Autodesk Inventor part; units mm, degrees
ref_plane "YZ Plane" through (0, 0, 0) normal (1, 0, 0) x (0, 1, 0)
ref_plane "XZ Plane" through (0, 0, 0) normal (0, 1, 0) x (-1, 0, 0)
ref_plane "XY Plane" through (0, 0, 0) normal (0, 0, 1) x (1, 0, 0)
sketch "Sketch1" plane through (0, 0, 0) normal (0, 0, 1) x (1, 0, 0)
  line L0 (0, 0) -> (20.32, 0)
  line L1 (20.32, 0) -> (20.32, -139.7)
  line L2 (20.32, -139.7) -> (0, -139.7)
  line L3 (0, -139.7) -> (0, 0)
  line L4 (0, 0) -> (7.62, 0)
  line L5 (20.32, 0) -> (12.7, 0)
  line L6 (7.62, 0) -> (7.62, -3.302)
  line L7 (12.7, 0) -> (12.7, -3.302)
  line L8 (12.7, -3.302) -> (17.78, -3.302)
  line L9 (17.78, -3.302) -> (17.78, -8.382)
  line L10 (17.78, -8.382) -> (12.7, -8.382)
  line L11 (12.7, -8.382) -> (12.7, -13.462)
  line L12 (12.7, -13.462) -> (7.62, -13.462)
  line L13 (7.62, -13.462) -> (7.62, -8.382)
  line L14 (7.62, -8.382) -> (2.54, -8.382)
  line L15 (2.54, -8.382) -> (2.54, -3.302)
  line L16 (2.54, -3.302) -> (7.62, -3.302)
  line L17 (7.62, -3.302) -> (7.62, 0)
  dimension "d0" = 20.32
  dimension "d1" = 139.7
  dimension "d2" = 7.62
  dimension "d3" = 7.62
  dimension "d4" = 3.302
  dimension "d5" = 5.08
  dimension "d6" = 5.08
  dimension "d7" = 5.08
  dimension "d8" = 5.08
  dimension "d9" = 5.08
  dimension "d10" = 5.08
  dimension "d11" = 5.08
  dimension "d12" = 5.08
  dimension "d13" = 5.08
extrude "Extrusion1" add sketch "Sketch1" along normal blind 13.97 contours L0 L6 L16 L15 L14 L13 L12 L11 L10 L9 L8 L7 L1 L2 L3
sketch "Sketch2" plane through (20.32, -139.7, 0) normal (1, 0, 0) x (0, 0, -1)
  line L0 (-10.7501, 15.4155) -> (-10.7501, 26.5915)
  line L1 (-10.7501, 26.5915) -> (-1.8601, 26.5915)
  line L2 (-1.8601, 26.5915) -> (-1.8601, 15.4155)
  line L3 (-1.8601, 15.4155) -> (-10.7501, 15.4155)
  line L4 (-10.7501, 65.6672) -> (-10.7501, 77.0972)
  line L5 (-10.7501, 77.0972) -> (-1.8601, 77.0972)
  line L6 (-1.8601, 77.0972) -> (-1.8601, 65.6672)
  line L7 (-1.8601, 65.6672) -> (-10.7501, 65.6672)
  point P0 (0, 139.7)
  dimension "d16" = 11.176
  dimension "d17" = 8.89
  dimension "d18" = 11.43
  dimension "d19" = 8.89
extrude "Extrusion2" cut sketch "Sketch2" against normal blind 533.4
shell "Shell1" thickness 6.35 removed faces 1 at (20.32, -20.8676, 8.24)
sketch "Sketch3" plane through (0, 0, 13.97) normal (0, 0, 1) x (1, 0, 0)
  point P0 (0, 0)
properties part number "ripnewvertical2"
Here's how the part is built. I have some questions about the finished solid (model axes, mm). A direction names the side the tool comes from. Give positions to 0.01 mm unless a question says otherwise; leave off trailing zeros. Write each loop counter-clockwise with the first axis right and the second up, starting at its lowest first coordinate (ties: lowest second). Pieces come first, ordered by that corner, then holes. Notation, with made-up numbers: (-40, 1) -> (-18, 1) arc R18 cw to (-18, 15) -> close; hole circle Ø6 at (52, 74). An arc over 180 degrees is marked (long way). Write each question's results on one line, items separated by ' | '.
Item 1: Suppose I cut it at B-B on z = 4.5. Write out the boundary of the cut face in (x, y).
Output:
outline: (0, -139.7) -> (20.32, -139.7) -> (20.32, -124.28) -> (0, -124.28) -> close; (0, -113.11) -> (20.32, -113.11) -> (20.32, -74.03) -> (0, -74.03) -> close; (0, -62.6) -> (20.32, -62.6) -> (20.32, 0) -> (12.7, 0) -> (12.7, -3.3) -> (17.78, -3.3) -> (17.78, -8.38) -> (12.7, -8.38) -> (12.7, -13.46) -> (7.62, -13.46) -> (7.62, -8.38) -> (2.54, -8.38) -> (2.54, -3.3) -> (7.62, -3.3) -> (7.62, 0) -> (0, 0) -> close
Item 2: Suppose I cut it at A-A on x = 15.75. Write out the boundary of the cut face in (y, z).
Output:
outline: (-139.7, 0) -> (-8.38, 0) -> (-8.38, 13.97) -> (-139.7, 13.97) -> close; (-3.3, 0) -> (0, 0) -> (0, 13.97) -> (-3.3, 13.97) -> close; hole (-133.35, 6.35) -> (-130.63, 6.35) -> (-130.63, 7.62) -> (-133.35, 7.62) -> close; hole (-124.28, 1.86) -> (-113.11, 1.86) -> (-113.11, 10.75) -> (-124.28, 10.75) -> close; hole (-106.76, 6.35) -> (-80.38, 6.35) -> (-80.38, 7.62) -> (-106.76, 7.62) -> close; hole (-74.03, 1.86) -> (-62.6, 1.86) -> (-62.6, 10.75) -> (-74.03, 10.75) -> close; hole (-56.25, 6.35) -> (-19.81, 6.35) -> (-19.81, 7.62) -> (-56.25, 7.62) -> close
Item 3: We'd pull the mould along X, two halves only. Please class faces 1 (the face through (7.62, -11, 7)), 2 (the face through (0, -71, 12)), 3 (the face through (2.54, -6, 7)), 4 (the face through (10, -139.7, 7)): pulls with the +X half, pulls with the -X half, needs draft (parallel to the pull), parting line crosses it, or undercut.
Output:
face 1: undercut | face 2: pulls with the -X half | face 3: undercut | face 4: needs draft
Item 4: If I drill on L1, parallel to Y at x = 16.25, z = 5.5; L2, parallel to Y at x = 1.75, z = 10.25; L3, parallel to Y at x = 12.25, z = 6, over which ranges is the centre line in solid material (lowest first)?
Output:
L1: y = -139.7 to -124.28, -113.11 to -74.03, -62.6 to -8.38, -3.3 to 0 | L2: y = -139.7 to -124.28, -113.11 to -74.03, -62.6 to 0 | L3: y = -139.7 to -124.28, -113.11 to -74.03, -62.6 to -13.46
Item 5: Suppose I cut it at D-D on x = 9. Write out the boundary of the cut face in (y, z), plus the area to 3 significant figures.
Output:
outline: (-139.7, 0) -> (-13.46, 0) -> (-13.46, 13.97) -> (-139.7, 13.97) -> close; hole (-133.35, 6.35) -> (-130.63, 6.35) -> (-130.63, 7.62) -> (-133.35, 7.62) -> close; hole (-124.28, 1.86) -> (-113.11, 1.86) -> (-113.11, 10.75) -> (-124.28, 10.75) -> close; hole (-106.76, 6.35) -> (-80.38, 6.35) -> (-80.38, 7.62) -> (-106.76, 7.62) -> close; hole (-74.03, 1.86) -> (-62.6, 1.86) -> (-62.6, 10.75) -> (-74.03, 10.75) -> close; hole (-56.25, 6.35) -> (-19.81, 6.35) -> (-19.81, 7.62) -> (-56.25, 7.62) -> close | area: 1,480 mm^2
Item 6: Suppose I cut it at C-C on y = -69. Write out the boundary of the cut face in (x, z).
Output:
outline: (0, 0) -> (20.32, 0) -> (20.32, 1.86) -> (0, 1.86) -> close; (0, 10.75) -> (20.32, 10.75) -> (20.32, 13.97) -> (0, 13.97) -> close
Item 7: For pin 1 Ø4 at (x, z) = (6.5, 11) entering from +Y; pin 2 Ø3 at (y, z) = (-64.5, 7.5) entering from -X; pin 3 Ø1 at (x, z) = (10, 6) entering from +Y, each with a flat end and sliding along its axis, tell me the tip position at first contact or that it passes through.
Output:
pin 1: stops at y = 0 | pin 2: passes through | pin 3: stops at y = -13.46
Item 8: On a 3-axis mill with a long thin cutter (end or side, diameter ignored), from which of +Z, -Z, +X, -X, +Y, -Y can I reach the whole of each face in a straight line? I mean faces 5 (the face through (17.78, -6, 7)), 6 (the face through (10, -113.108, 6)), 7 (the face through (7.62, -2, 7)), 8 (the face through (13, -93, 7.62)). Say none if no direction works.
Output:
face 5: +Z, -Z | face 6: +X, -X | face 7: +Z, -Z, +Y | face 8: +X
